```python
from build123d import *

# Parameters (mm, degrees)
BOSS_EXTRUDE1_DEPTH      = 3.175
SKETCH2_R                = 16.9545
CUT_EXTRUDE1_DEPTH       = 600.06621556
CONVERT_SOLID1_START     = -1.5875
CONVERT_SOLID1_OUTLINE_R = 16.9545
CONVERT_SOLID1_DEPTH     = 1.5875
EDGE_FLANGE3_DEPTH       = 19.05
SKETCH17_R               = 3.302
CUT_EXTRUDE4_DEPTH       = 609.89886437
CUT_EXTRUDE5_DEPTH       = 609.89886437
SKETCH19_R               = 3.302
CUT_EXTRUDE6_DEPTH       = 610.147146247


# Read off the part's stored shape, not the designer's step: Convert-Solid1
# Sheet-metal steps are written as plain solids
with BuildPart() as part:
    # Sketch1 → Boss-Extrude1 (new body)
    with BuildSketch(Plane.XY):
        with BuildLine():
            Line((6.35, 0), (317.5, 0))
            Line((317.5, 0), (317.5, 25.4))
            Line((317.5, 25.4), (181.457249023, 52.608550195))
            ThreePointArc((181.457249023, 52.608550195), (140.315142877, 75.746018143), (120.694108864, 118.676547437))
            Line((120.694108864, 118.676547437), (76.2, 508))
            Line((76.2, 508), (6.35, 508))
            ThreePointArc((6.35, 508), (1.859871939, 506.140128061), (0, 501.65))
            Line((0, 501.65), (0, 6.35))
            ThreePointArc((0, 6.35), (1.859871939, 1.859871939), (6.35, 0))
        make_face()
    extrude(amount=BOSS_EXTRUDE1_DEPTH)

    # Sketch2 → Cut-Extrude1 (cut, through all)
    with BuildSketch(Plane.XY.offset(3.175)):
        with Locations((20.574, 486.9942)):
            Circle(SKETCH2_R)
        with Locations((20.574, 20.574)):
            Circle(SKETCH2_R)
    extrude(amount=-CUT_EXTRUDE1_DEPTH, mode=Mode.SUBTRACT)

    # Convert-Solid1 outline → Convert-Solid1 (add)
    with BuildSketch(Plane.XY.offset(CONVERT_SOLID1_START)):
        with BuildLine():
            Line((317.5, 25.4), (181.457249023, 52.608550195))
            ThreePointArc((181.457249023, 52.608550195), (140.315142877, 75.746018143), (120.694108864, 118.676547437))
            Line((120.694108864, 118.676547437), (76.2, 508))
            Line((76.2, 508), (6.35, 508))
            ThreePointArc((6.35, 508), (1.859871939, 506.140128061), (0, 501.65))
            Line((0, 501.65), (0, 6.35))
            ThreePointArc((0, 6.35), (1.859871939, 1.859871939), (6.35, 0))
            Line((6.35, 0), (317.5, 0))
            Line((317.5, 0), (317.5, 25.4))
        make_face()
        with Locations((20.574, 20.574)):
            Circle(CONVERT_SOLID1_OUTLINE_R, mode=Mode.SUBTRACT)
        with Locations((20.574, 486.9942)):
            Circle(CONVERT_SOLID1_OUTLINE_R, mode=Mode.SUBTRACT)
    extrude(amount=CONVERT_SOLID1_DEPTH)

    # Edge-Flange3 section (across the edge) → Edge-Flange3 (add)
    with BuildSketch(Plane(origin=(76.2, 512.7625, 3.175), x_dir=(0, -1, 0), z_dir=(-1, 0, 0))):
        with BuildLine():
            Line((-4.7625, 4.7625), (-4.7625, 46.0375))
            Line((-4.7625, 46.0375), (0, 46.0375))
            Line((0, 46.0375), (0, 4.7625))
            ThreePointArc((0, 4.7625), (1.394903955, 1.394903955), (4.7625, 0))
            Line((4.7625, 0), (4.7625, -4.7625))
            ThreePointArc((4.7625, -4.7625), (-1.972692091, -1.972692091), (-4.7625, 4.7625))
        make_face()
    extrude(amount=EDGE_FLANGE3_DEPTH)

    # Sketch17 → Cut-Extrude4 (cut, through all)
    with BuildSketch(Plane.XY.offset(3.175)):
        with Locations((76.2, 423.892006342)):
            Circle(SKETCH17_R)
        with Locations((76.2, 347.692006342)):
            Circle(SKETCH17_R)
        with Locations((76.2, 271.492006342)):
            Circle(SKETCH17_R)
        with Locations((76.2, 195.292006342)):
            Circle(SKETCH17_R)
        with Locations((76.2, 119.092006342)):
            Circle(SKETCH17_R)
        with Locations((266.7, 22.225)):
            Circle(SKETCH17_R)
        with Locations((165.1, 22.225)):
            Circle(SKETCH17_R)
    extrude(amount=-CUT_EXTRUDE4_DEPTH, mode=Mode.SUBTRACT)

    # Sketch18 → Cut-Extrude5 (cut, through all)
    with BuildSketch(Plane.XY.offset(3.175)):
        with BuildLine():
            Line((3.6195, 28.2067), (3.6195, 20.574))
            ThreePointArc((3.6195, 20.574), (20.574, 3.6195), (37.5285, 20.574))
            Line((37.5285, 20.574), (37.5285, 28.2067))
            ThreePointArc((37.5285, 28.2067), (20.574, 45.1612), (3.6195, 28.2067))
        make_face()
    extrude(amount=-CUT_EXTRUDE5_DEPTH, mode=Mode.SUBTRACT)

    # Sketch19 → Cut-Extrude6 (cut, through all)
    with BuildSketch(Plane(origin=(0, 517.525, 0), x_dir=(0, 0, -1), z_dir=(0, 1, 0))):
        with Locations((-28.575, -82.55)):
            Circle(SKETCH19_R)
        with Locations((-28.575, -50.8)):
            Circle(SKETCH19_R)
    extrude(amount=-CUT_EXTRUDE6_DEPTH, mode=Mode.SUBTRACT)


solid = part.part
```
Build history of the part. All positions in model axes, mm. A direction names the side the tool comes from. Give positions to 0.01 mm unless a question says otherwise; leave off trailing zeros. Loops run counter-clockwise (first coordinate to the right, second up) from the corner with the lowest first, then second, coordinate; pieces in that order, holes last. Notation, with made-up numbers: (-26, -21) - (-15, -21) arc R30 ccw to (-15, 9) - close; hole circle Ø2 at (-22.75, 2). An arc over 180 degrees is marked (long way). Use a Markdown table: item, result.
(1) Drop flat-ended pins along their axis: pin 1 Ø10.5 at (x, y) = (76.2, 271.49) entering from +Z (3 decimals); pin 2 Ø4 at (x, y) = (76.2, 119.09) entering from +Z; pin 3 Ø3 at (y, z) = (514, 21.5) entering from +X; pin 4 Ø21 at (x, z) = (67, 18.5) entering from -Y. Give the stop position or say it passes through.
Taken from the geometry:
| item | result |
|---|---|
| pin 1 | z = 3.175 |
| pin 2 | through |
| pin 3 | x = 76.2 |
| pin 4 | y = 512.76 |
(2) Wall check: line 1 along Z through (x, y) = (61.5, 194.5) (1 decimal); line 2 along Y through (x, z) = (58, 13.5) (1 decimal); line 3 along Y through (x, z) = (47.5, 3). Give the ranges that are in metal, low to high.
Taken from the geometry:
| item | result |
|---|---|
| line 1 | -1.6 to 3.2 |
| line 2 | 512.8 to 517.5 |
| line 3 | 0 to 508 |
(3) Which spindle directions (+Z, -Z, +X, -X, +Y, -Y) get a long thin tool onto all of the face, cutting with end or side? Do faces 1 (the face through (76, 199, 3.175)), 2 (the face through (20.201, 3.624, 0.76)), 3 (the face through (76.2, 515, 24)), 4 (the face through (57.15, 515, 24)), 5 (the face through (76, 199, -1.588)). Say none if no direction does.
Taken from the geometry:
| item | result |
|---|---|
| face 1 | +Z, +X, -X, -Y |
| face 2 | +Z, -Z |
| face 3 | +Z, -Z, +X, +Y |
| face 4 | +Z, -Z, -X, +Y |
| face 5 | -Z, +X, -X, +Y, -Y |
(4) Pull direction X, two halves, no side cores. Call faces 6 (the face through (20.947, 45.157, 0.827)), 7 (the face through (98.76, 310.61, 0.76)), 8 (the face through (67, 517.525, 28)): +X half, -X half, draft (parallel to the pull), parting line (faces both ways), or undercut.
Taken from the geometry:
| item | result |
|---|---|
| face 6 | undercut |
| face 7 | +X half |
| face 8 | draft |
(5) Band-saw the part on A-A (y = 228). Give the cut face in (x, z) (1 decimal).
Taken from the geometry:
| item | result |
|---|---|
| outline | (0, -1.6) - (108.2, -1.6) - (108.2, 3.2) - (0, 3.2) - close |
